```python
from build123d import *

# Parameters (mm, degrees)
SKETCH13_R          = 40
BOSS_EXTRUDE1_DEPTH = 1000


with BuildPart() as part:
    # Sketch13 → Boss-Extrude1 (new body)
    with BuildSketch(Plane.XY):
        with BuildLine():
            Line((51.91795422, 36.025866242), (-161.747997967, 196.755140095))
            ThreePointArc((-161.747997967, 196.755140095), (-194.454364826, 194.454364826), (-196.755140095, 161.747997967))
            Line((-196.755140095, 161.747997967), (-47.948267516, -36.068873592))
            ThreePointArc((-47.948267516, -36.068873592), (-2.54296529, -59.946086841), (44.72135955, -40))
            ThreePointArc((44.72135955, -40), (54.834590611, -32.613872125), (67.082039325, -30))
            Line((67.082039325, -30), (232.917960675, -30))
            ThreePointArc((232.917960675, -30), (245.165409389, -32.613872125), (255.27864045, -40))
            ThreePointArc((255.27864045, -40), (360, 0), (255.27864045, 40))
            ThreePointArc((255.27864045, 40), (245.165409389, 32.613872125), (232.917960675, 30))
            Line((232.917960675, 30), (69.952391016, 30))
            ThreePointArc((69.952391016, 30), (60.445130968, 31.546318228), (51.91795422, 36.025866242))
        make_face()
        with Locations((300, 0)):
            Circle(SKETCH13_R, mode=Mode.SUBTRACT)
        with BuildLine():
            Line((-10.606601718, -10.606601718), (-187.383297014, 166.170093579))
            ThreePointArc((-187.383297014, 166.170093579), (-187.383297014, 187.383297014), (-166.170093579, 187.383297014))
            Line((-166.170093579, 187.383297014), (10.606601718, 10.606601718))
            ThreePointArc((10.606601718, 10.606601718), (10.606601718, -10.606601718), (-10.606601718, -10.606601718))
        make_face(mode=Mode.SUBTRACT)
    extrude(amount=BOSS_EXTRUDE1_DEPTH)


solid = part.part
```
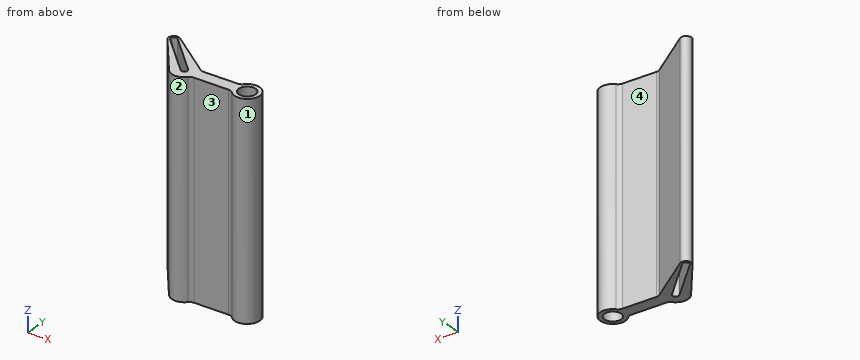
For this review, take the finished solid that the model builds, in its own axes (mm). Face numbers are marked on the shaded views. A direction names the side the tool comes from. Coordinates: 2 decimals unless noted, no trailing zeros. Loops run counter-clockwise (first coordinate to the right, second up) from the corner with the lowest first, then second, coordinate; pieces in that order, holes last. Notation, with made-up numbers: (10.25, 67) -> (23.25, 67) arc R6 ccw to (23.25, 74) -> close; hole circle Ø9 at (-27.5, -14.75). An arc over 180 degrees is marked (long way). Return JSON: item names as keys, results as strings. Group by question number.
(1) For pin 1 Ø3 at (x, z) = (189.5, 865.5) entering from +Y; pin 2 Ø12 at (y, z) = (3.5, 552.5) entering from -X; pin 3 Ø5 at (x, z) = (-13, 189) entering from +Y, all flat-tipped, find the tip position at first contact; note any pin that passes through.
(2) Consider section C-C, the plane z = 443.5. Give the boundary of the cut face in (x, y), plus the area to 3 significant figures.
(3) To check wall thickness, follow L1, parallel to X at y = -12, z = 881; L2, parallel to X at y = -33.5, z = 782.5; L3, parallel to Y at x = 300, z = 721. State the ranges of each line that lie inside material, in increasing order.
(4) Mouldability with a two-part tool opening along X and no side actions: class the marked faces 1 and 2 as pulls with the +X half, pulls with the -X half, needs draft (parallel to the pull), parting line crosses it, or undercut.
(5) Tool access review of the marked faces 3 and 4: name each direction out of +Z, -Z, +X, -X, +Y, -Y from which nothing blocks a thin tool from reaching the whole face with its end or side.
(6) Consider section B-B, the plane x = 300. Give the boundary of the cut face in (y, z), plus the area to 3 significant figures.
(7) Consider section A-A, the plane y = 117. Give the boundary of the cut face in (x, z), plus the area to 3 significant figures.
(8) Consider section D-D, the plane y = 0. Give the boundary of the cut face in (x, z).
Results below:
{
 "1": {"pin 1": "stops at y = 30", "pin 2": "stops at x = -82.23", "pin 3": "stops at y = 86.74"},
 "2": {"outline": "(-196.76, 161.75) -> (-47.95, -36.07) arc R60 ccw to (44.72, -40) arc R30 cw to (67.08, -30) -> (232.92, -30) arc R30 cw to (255.28, -40) arc R60 ccw (long way) to (255.28, 40) arc R30 cw to (232.92, 30) -> (69.95, 30) arc R30 cw to (51.92, 36.03) -> (-161.75, 196.76) arc R25 ccw to start; hole (-187.38, 166.17) -> (-10.61, -10.61) arc R15 ccw to (10.61, 10.61) -> (-166.17, 187.38) arc R15 ccw to start; hole circle Ø80 at (300, 0)", "area": "37,400 mm2"},
 "3": {"L1": "x = -66.05 to -9, 9 to 261.84, 338.16 to 358.79", "L2": "x = -49.88 to 53.02, 246.98 to 278.14, 321.86 to 349.78", "L3": "y = -60 to -40, 40 to 60"},
 "4": {"face 1": "undercut", "face 2": "undercut"},
 "5": {"face 3": "+Z, -Z, -Y", "face 4": "+Z, -Z, +Y"},
 "6": {"outline": "(-60, 0) -> (-40, 0) -> (-40, 1000) -> (-60, 1000) -> close; (40, 0) -> (60, 0) -> (60, 1000) -> (40, 1000) -> close", "area": "40,000 mm2"},
 "7": {"outline": "(-163.09, 0) -> (-138.21, 0) -> (-138.21, 1000) -> (-163.09, 1000) -> close; (-95.79, 0) -> (-55.73, 0) -> (-55.73, 1000) -> (-95.79, 1000) -> close", "area": "64,900 mm2"},
 "8": {"outline": "(-75.08, 0) -> (-21.21, 0) -> (-21.21, 1000) -> (-75.08, 1000) -> close; (15, 0) -> (260, 0) -> (260, 1000) -> (15, 1000) -> close; (340, 0) -> (360, 0) -> (360, 1000) -> (340, 1000) -> close"}
}
